Read the model definition and answer for the solid it produces. Units are mm, in the model's axes. Round coordinates to 2 decimals unless told otherwise and drop trailing zeros. Write each loop counter-clockwise with the first axis right and the second up, starting at its lowest first coordinate (ties: lowest second). Pieces come first, ordered by that corner, then holes.
from build123d import *

# Parameters (mm, degrees)
SKETCH1_W           = 160
SKETCH1_H           = 136.35
SKETCH1_R           = 11.25
SKETCH1_W_2         = 10
SKETCH1_H_2         = 3.175
SKETCH1_W_3         = 3.175
SKETCH1_H_3         = 10
BOSS_EXTRUDE1_DEPTH = 3.175


with BuildPart() as part:
    # Sketch1 → Boss-Extrude1 (new body)
    with BuildSketch(Plane.XY):
        with Locations((80, 68.069958461)):
            Rectangle(SKETCH1_W, SKETCH1_H)
        with Locations((80, 68.069958461)):
            Circle(SKETCH1_R, mode=Mode.SUBTRACT)
        with Locations((40, 131.482458461)):
            Rectangle(SKETCH1_W_2, SKETCH1_H_2, mode=Mode.SUBTRACT)
        with Locations((20, 131.482458461)):
            Rectangle(SKETCH1_W_2, SKETCH1_H_2, mode=Mode.SUBTRACT)
        with Locations((60, 131.482458461)):
            Rectangle(SKETCH1_W_2, SKETCH1_H_2, mode=Mode.SUBTRACT)
        with Locations((80, 131.482458461)):
            Rectangle(SKETCH1_W_2, SKETCH1_H_2, mode=Mode.SUBTRACT)
        with Locations((100, 131.482458461)):
            Rectangle(SKETCH1_W_2, SKETCH1_H_2, mode=Mode.SUBTRACT)
        with Locations((120, 131.482458461)):
            Rectangle(SKETCH1_W_2, SKETCH1_H_2, mode=Mode.SUBTRACT)
        with Locations((140, 131.482458461)):
            Rectangle(SKETCH1_W_2, SKETCH1_H_2, mode=Mode.SUBTRACT)
        with Locations((140, 4.657458461)):
            Rectangle(SKETCH1_W_2, SKETCH1_H_2, mode=Mode.SUBTRACT)
        with Locations((120, 4.657458461)):
            Rectangle(SKETCH1_W_2, SKETCH1_H_2, mode=Mode.SUBTRACT)
        with Locations((100, 4.657458461)):
            Rectangle(SKETCH1_W_2, SKETCH1_H_2, mode=Mode.SUBTRACT)
        with Locations((80, 4.657458461)):
            Rectangle(SKETCH1_W_2, SKETCH1_H_2, mode=Mode.SUBTRACT)
        with Locations((60, 4.657458461)):
            Rectangle(SKETCH1_W_2, SKETCH1_H_2, mode=Mode.SUBTRACT)
        with Locations((40, 4.657458461)):
            Rectangle(SKETCH1_W_2, SKETCH1_H_2, mode=Mode.SUBTRACT)
        with Locations((20, 4.657458461)):
            Rectangle(SKETCH1_W_2, SKETCH1_H_2, mode=Mode.SUBTRACT)
        with Locations((4.5875, 38.069958461)):
            Rectangle(SKETCH1_W_3, SKETCH1_H_3, mode=Mode.SUBTRACT)
        with Locations((4.5875, 98.069958461)):
            Rectangle(SKETCH1_W_3, SKETCH1_H_3, mode=Mode.SUBTRACT)
        with Locations((4.5875, 118.069958461)):
            Rectangle(SKETCH1_W_3, SKETCH1_H_3, mode=Mode.SUBTRACT)
        with Locations((4.5875, 18.069958461)):
            Rectangle(SKETCH1_W_3, SKETCH1_H_3, mode=Mode.SUBTRACT)
        with Locations((155.4125, 18.069958461)):
            Rectangle(SKETCH1_W_3, SKETCH1_H_3, mode=Mode.SUBTRACT)
        with Locations((155.4125, 38.069958461)):
            Rectangle(SKETCH1_W_3, SKETCH1_H_3, mode=Mode.SUBTRACT)
        with Locations((155.4125, 98.069958461)):
            Rectangle(SKETCH1_W_3, SKETCH1_H_3, mode=Mode.SUBTRACT)
        with Locations((155.4125, 118.069958461)):
            Rectangle(SKETCH1_W_3, SKETCH1_H_3, mode=Mode.SUBTRACT)
    extrude(amount=BOSS_EXTRUDE1_DEPTH)


solid = part.part
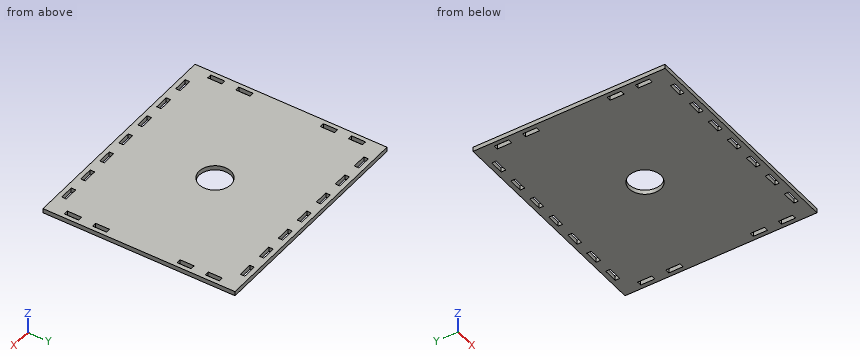
Q1. Straight lines are drawn through the part: probe 1 along Y at (x, z) = (80, 1.55); probe 2 along Y at (x, z) = (16.5, 2.65); probe 3 along X at (y, z) = (40.5, 1.2) (3 decimals). For each, find the intervals that lie inside material, in ascending order.
Verdict:
probe 1: y = -0.11 to 3.07, 6.24 to 56.82, 79.32 to 129.89, 133.07 to 136.24
probe 2: y = -0.11 to 3.07, 6.24 to 129.89, 133.07 to 136.24
probe 3: x = 0 to 3, 6.175 to 153.825, 157 to 160
Q2. Section A-A (x = 80) is taken. Determine the outline of the cut face in (y, z) (3 decimals), then the cut area to 3 significant figures.
Verdict:
outline: (-0.105, 0) - (3.07, 0) - (3.07, 3.175) - (-0.105, 3.175) - close; (6.245, 0) - (56.82, 0) - (56.82, 3.175) - (6.245, 3.175) - close; (79.32, 0) - (129.895, 0) - (129.895, 3.175) - (79.32, 3.175) - close; (133.07, 0) - (136.245, 0) - (136.245, 3.175) - (133.07, 3.175) - close
area: 341 mm2
Q3. Section B-B (y = 40) is taken. Determine the outline of the cut face in (x, z) (3 decimals), then the cut area to 3 significant figures.
Verdict:
outline: (0, 0) - (3, 0) - (3, 3.175) - (0, 3.175) - close; (6.175, 0) - (153.825, 0) - (153.825, 3.175) - (6.175, 3.175) - close; (157, 0) - (160, 0) - (160, 3.175) - (157, 3.175) - close
area: 488 mm2
Q4. Section C-C (z = 2.1) is taken. State how many separate pieces and enclosed holes the cut face has, then the cut area to 3 significant figures.
Verdict:
separate pieces: 1
enclosed holes: 23
area: 20,700 mm2
